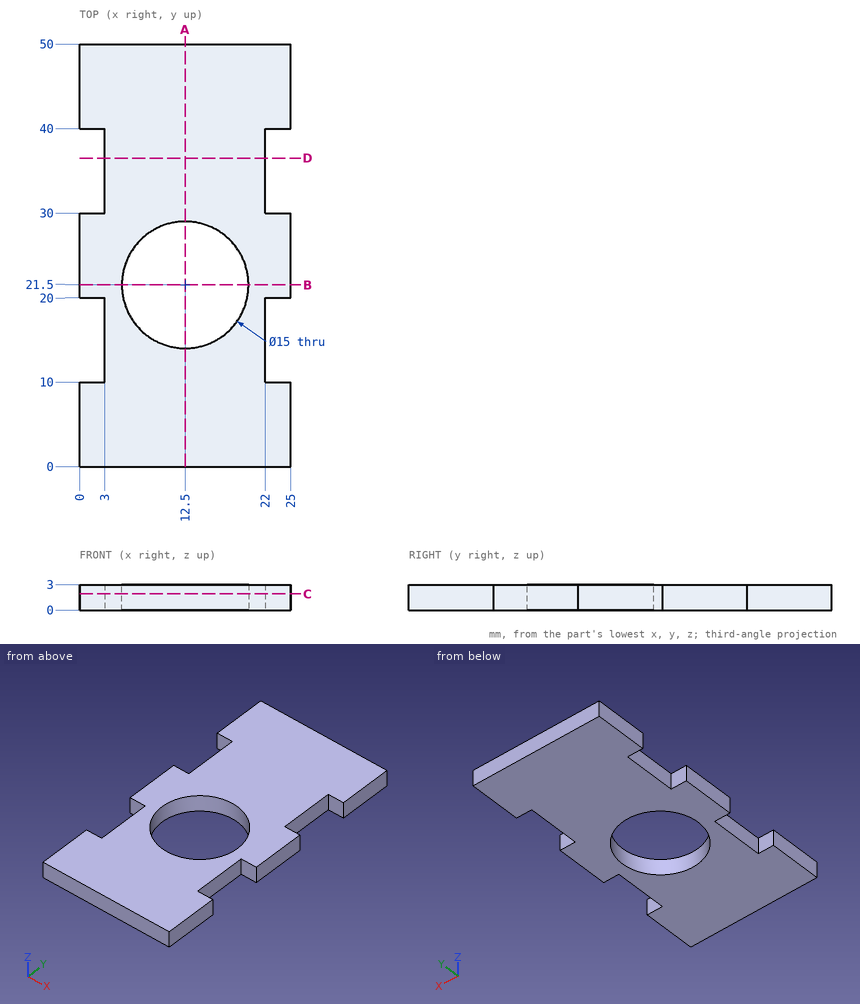
Can you work these out from the drawing? Everything is in mm from the part's minimum corner. Round coordinates to 2 decimals unless told otherwise and drop trailing zeros. Loops run counter-clockwise (first coordinate to the right, second up) from the corner with the lowest first, then second, coordinate; pieces in that order, holes last.
1. For P1, Ø0.9, axis at y = 16, z = 1.5, coming from the -X side; P2, Ø0.9, axis at x = 1, z = 2, coming from the -Y side; P3, Ø1.5, axis at y = 14.5, z = 1, coming from the +X side, each with a flat end and sliding along its axis, tell me the tip position at first contact or that it passes through.
Answer list:
P1: stops at x = 3
P2: stops at y = 0
P3: stops at x = 22
2. If I drill on line 1 along Y through (x, z) = (2.25, 1.7); line 2 along Y through (x, z) = (12.5, 0.8); line 3 along X through (y, z) = (34, 0.7), over which ranges is the centre line in solid material (lowest first)?
Answer list:
line 1: y = 0 to 10, 20 to 30, 40 to 50
line 2: y = 0 to 14, 29 to 50
line 3: x = 3 to 22
3. If we section it at A-A on x = 12.5: Write out the boundary of the cut face in (y, z), plus the area to 3 significant figures.
Answer list:
outline: (0, 0) - (14, 0) - (14, 3) - (0, 3) - close; (29, 0) - (50, 0) - (50, 3) - (29, 3) - close
area: 105 mm2
4. If we section it at D-D on y = 36.5: Write out the boundary of the cut face in (x, z).
Answer list:
outline: (3, 0) - (22, 0) - (22, 3) - (3, 3) - close
5. If we section it at B-B on y = 21.5: Write out the boundary of the cut face in (x, z), plus the area to 3 significant figures.
Answer list:
outline: (0, 0) - (5, 0) - (5, 3) - (0, 3) - close; (20, 0) - (25, 0) - (25, 3) - (20, 3) - close
area: 30.0 mm2
6. If we section it at C-C on z = 1.9: Write out the boundary of the cut face in (x, y), plus the area to 3 significant figures.
Answer list:
outline: (0, 0) - (25, 0) - (25, 10) - (22, 10) - (22, 20) - (25, 20) - (25, 30) - (22, 30) - (22, 40) - (25, 40) - (25, 50) - (0, 50) - (0, 40) - (3, 40) - (3, 30) - (0, 30) - (0, 20) - (3, 20) - (3, 10) - (0, 10) - close; hole circle Ø15 at (12.5, 21.5)
area: 953 mm2
